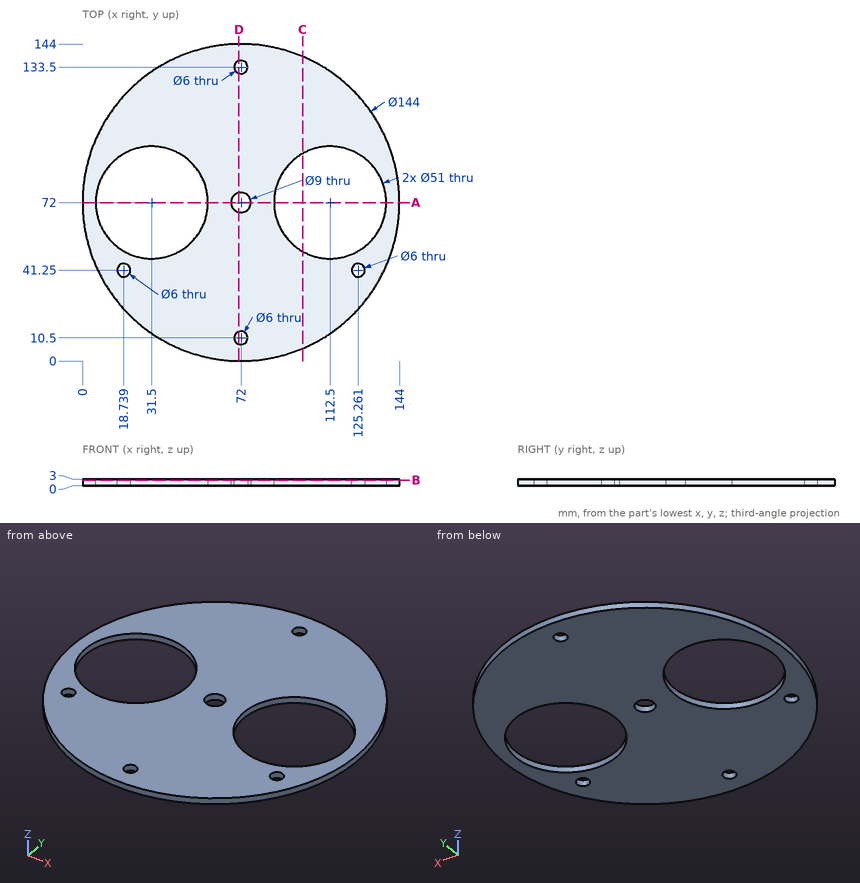
Here's the drawing with two shaded views (mm, measured from the low corner). I have some questions. Give positions to 0.01 mm unless a question says otherwise; leave off trailing zeros. Write each loop counter-clockwise with the first axis right and the second up, starting at its lowest first coordinate (ties: lowest second). Pieces come first, ordered by that corner, then holes. Notation, with made-up numbers: (30, 53.5) -> (59, 53.5) arc R9 ccw to (59, 65.5) -> close; hole circle Ø11 at (29.25, 42). An arc over 180 degrees is marked (long way). Answer as a JSON object with one key per item and string values. Group by question number.
Item 1: Suppose I cut it at D-D (x = 71). Please give me the cut outline in (y, z).
Item 2: I'm going to push flat-ended pins straight in: P1, Ø1.5, axis at x = 47.5, z = 0.5, coming from the +Y side; P2, Ø1.5, axis at y = 61.5, z = 0.5, coming from the +X side. Where does each tip first touch, or does it pass through?
Item 3: Please list where these lines run through material, in increasing order: line 1 (Y direction, x = 72, z = 2.2); line 2 (X direction, y = 61, z = 1) (1 decimal); line 3 (X direction, y = 77.5, z = 0.65). Write a range as [from, to].
Item 4: Suppose I cut it at B-B (z = 2.45). Please give me the cut outline in (x, y), plus the area to 3 significant figures.
Item 5: Suppose I cut it at C-C (x = 100). Please give me the cut outline in (y, z).
Item 6: Suppose I cut it at A-A (y = 72). Please give me the cut outline in (x, z).
Findings:
{
 "1": {"outline": "(0.01, 0) -> (7.67, 0) -> (7.67, 3) -> (0.01, 3) -> close; (13.33, 0) -> (67.61, 0) -> (67.61, 3) -> (13.33, 3) -> close; (76.39, 0) -> (130.67, 0) -> (130.67, 3) -> (76.39, 3) -> close; (136.33, 0) -> (143.99, 0) -> (143.99, 3) -> (136.33, 3) -> close"},
 "2": {"P1": "stops at y = 139.97", "P2": "stops at x = 143.34"},
 "3": {"line 1": "y = [0, 7.5], [13.5, 67.5], [76.5, 130.5], [136.5, 144]", "line 2": "x = [0.8, 8.5], [54.5, 89.5], [135.5, 143.2]", "line 3": "x = [0.21, 6.6], [56.4, 87.6], [137.4, 143.79]"},
 "4": {"outline": "circle Ø144 at (72, 72); hole circle Ø51 at (31.5, 72); hole circle Ø6 at (18.74, 41.25); hole circle Ø9 at (72, 72); hole circle Ø6 at (72, 10.5); hole circle Ø6 at (72, 133.5); hole circle Ø51 at (112.5, 72); hole circle Ø6 at (125.26, 41.25)", "area": "12,000 mm²"},
 "5": {"outline": "(5.67, 0) -> (49.77, 0) -> (49.77, 3) -> (5.67, 3) -> close; (94.23, 0) -> (138.33, 0) -> (138.33, 3) -> (94.23, 3) -> close"},
 "6": {"outline": "(0, 0) -> (6, 0) -> (6, 3) -> (0, 3) -> close; (57, 0) -> (67.5, 0) -> (67.5, 3) -> (57, 3) -> close; (76.5, 0) -> (87, 0) -> (87, 3) -> (76.5, 3) -> close; (138, 0) -> (144, 0) -> (144, 3) -> (138, 3) -> close"}
}
